Check sheet for the modelled part. Datum: model origin and axes. Units: mm. Face numbers are marked on the shaded views. A direction names the side the tool comes from. Round coordinates to 2 decimals unless told otherwise and drop trailing zeros.
Item 1: Material ranges on line 1 along Y through (x, z) = (0, 5.3); line 2 along Y through (x, z) = (-4, 1.1); line 3 along Y through (x, z) = (3.5, 0.4), recorded low to high.
Item 2: Release check for a two-part mould opening along Y. For the marked faces 1, 2, 3 and 4 record: pulls with the +Y half, pulls with the -Y half, needs draft (parallel to the pull), parting line crosses it, or undercut.
Item 3: Set-up check for the marked faces 5 and 6: record each of +Z, -Z, +X, -X, +Y, -Y from which the full face is reachable in a straight line by a thin tool's end or side.
Item 4: Depth check by flat-ended pin: pin 1 (1.2 mm diameter, centred on x = -3.5, z = 1, fed in from -Y); pin 2 (6 mm diameter, centred on x = -3, y = -5, fed in from -Z); pin 3 (3 mm diameter, centred on y = 5, z = 4, fed in from -X); pin 4 (1.2 mm diameter, centred on y = 4.5, z = 0.5, fed in from -X). Enter the tip coordinate at first touch or a pass-through.
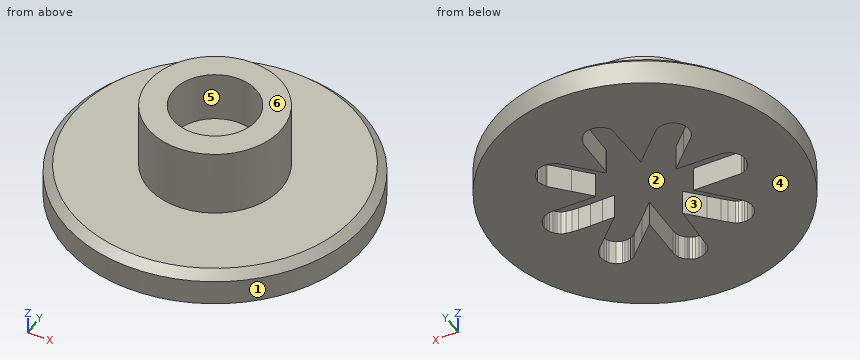
from build123d import *

# Parameters (mm, degrees)
F0_R     = 9
F1_DEPTH = 2
F2_R     = 4
F3_DEPTH = 4
F4_R     = 2.5
F5_DEPTH = 3
F6_SIZE  = 0.5
F8_DEPTH = 1.5


with BuildPart() as f1:
    # F0 (on Top) → F1 (new body)
    with BuildSketch(Plane.XY):
        Circle(F0_R)
    extrude(amount=F1_DEPTH)

    # F2 (on face) → F3 (join)
    with BuildSketch(Plane.XY.offset(2)):
        Circle(F2_R)
    extrude(amount=F3_DEPTH)

    # F4 (on face) → F5 (cut)
    with BuildSketch(Plane.XY.offset(6)):
        Circle(F4_R)
    extrude(amount=-F5_DEPTH, mode=Mode.SUBTRACT)

    # F6
    f6_edges = [f1.edges().sort_by_distance(p)[0] for p in [
        (-9, 0, 2),
    ]]
    chamfer(f6_edges, length=F6_SIZE)

    # F7 (on face) → F8 (cut)
    with BuildSketch(Plane(origin=(0, 0, 0), x_dir=(1, 0, 0), z_dir=(0, 0, -1))):
        Polygon((-0.031379, 5.948377), (-0.235333, 5.919157), (-0.372759, 5.868757), (-0.500818, 5.801363), (-0.64831, 5.683569), (-0.711513, 5.643549), (-0.766303, 5.595223), (-0.884297, 5.389084), (-0.972792, 2.355883), (-1.91674, 3.298237), (-2.464657, 3.842872), (-2.74588, 4.106761), (-3.037677, 4.358384), (-3.197437, 4.424921), (-3.362159, 4.476179), (-3.5244, 4.487041), (-3.686641, 4.476179), (-4.011123, 4.358384), (-4.276609, 4.122796), (-4.349034, 4.030994), (-4.401972, 3.928468), (-4.483097, 3.710516), (-4.483097, 3.357134), (-4.394602, 3.092097), (-4.24711, 2.885957), (-3.303163, 1.914155), (-2.359215, 0.971802), (-5.220556, 0.942353), (-5.397547, 0.883456), (-5.427045, 0.854008), (-5.556038, 0.793243), (-5.614945, 0.756011), (-5.663032, 0.706765), (-5.840022, 0.471176), (-5.958016, 0.117794), (-5.958016, -0.058897), (-5.940408, -0.209293), (-5.899019, -0.353383), (-5.843566, -0.461413), (-5.781025, -0.559523), (-5.655249, -0.699811), (-5.51554, -0.82456), (-5.220556, -0.942354), (-5.075648, -0.968558), (-4.928112, -0.97628), (-4.630589, -0.971802), (-4.188114, -0.971802), (-2.359215, -0.971802), (-2.368134, -1.005446), (-2.388713, -1.030699), (-3.332661, -1.973053), (-4.276609, -2.915406), (-4.34313, -2.999393), (-4.394602, -3.092097), (-4.419005, -3.155066), (-4.453599, -3.209892), (-4.476923, -3.415726), (-4.483097, -3.622171), (-4.464349, -3.757662), (-4.424101, -3.887208), (-4.374765, -3.997645), (-4.306107, -4.093348), (-4.188114, -4.240591), (-4.103985, -4.307), (-4.011123, -4.358385), (-3.71614, -4.476179), (-3.391658, -4.476179), (-3.067176, -4.387833), (-2.890186, -4.240591), (-1.946238, -3.298237), (-1.00229, -2.355884), (-0.884297, -5.418533), (-0.8253, -5.506878), (-0.699524, -5.647167), (-0.559815, -5.771915), (-0.503448, -5.807594), (-0.441821, -5.830812), (-0.341941, -5.885287), (-0.235333, -5.919158), (0.089149, -5.948606), (0.384133, -5.889709), (0.708615, -5.654121), (0.754319, -5.61094), (0.790702, -5.558969), (0.856107, -5.447981), (0.9741, -5.094599), (0.9741, -4.417282), (0.9741, -2.591472), (0.971489, -2.477691), (0.979459, -2.426523), (1.003599, -2.385332), (1.947546, -3.327686), (2.891494, -4.270039), (3.122896, -4.385014), (3.363468, -4.476179), (3.68795, -4.476179), (3.805943, -4.446731), (3.94337, -4.39633), (4.071429, -4.328936), (4.218921, -4.211142), (4.425409, -3.916657), (4.513904, -3.474929), (4.444862, -3.229831), (4.398065, -3.113042), (4.336914, -3.003752), (4.300041, -2.947904), (4.277917, -2.885958), (3.33397, -1.943604), (2.390022, -1.001251), (2.41952, -0.971802), (2.861996, -0.971802), (4.690894, -0.971802), (4.972609, -0.968567), (5.251363, -0.942354), (5.280862, -0.912905), (5.546347, -0.82456), (5.723337, -0.61842), (5.839817, -0.478169), (5.883167, -0.404005), (5.900327, -0.323934), (5.934856, -0.237188), (5.954737, -0.147151), (5.958016, 0.039233), (5.925076, 0.228087), (5.870829, 0.412279), (5.7562, 0.594983), (5.685681, 0.672036), (5.605344, 0.736213), (5.428354, 0.883456), (5.192367, 0.942353), (4.838344, 0.987761), (4.482387, 1.011028), (3.766457, 1.011578), (3.048146, 0.984877), (2.331025, 0.971802), (3.274973, 1.914155), (4.218921, 2.856509), (4.337268, 2.979647), (4.379451, 3.047229), (4.395911, 3.121546), (4.454907, 3.209891), (4.513904, 3.504377), (4.444233, 3.827854), (4.386266, 3.98061), (4.307416, 4.122796), (4.04193, 4.358384), (3.717448, 4.476179), (3.555567, 4.481563), (3.392966, 4.476179), (3.215976, 4.44673), (3.186478, 4.417282), (3.038986, 4.358384), (2.944209, 4.294123), (2.861996, 4.211142), (1.918048, 3.268788), (0.9741, 2.326435), (0.9741, 3.092097), (0.9741, 4.947355), (0.94889, 5.186814), (0.885605, 5.418532), (0.649618, 5.713018), (0.576669, 5.769819), (0.540299, 5.792295), (0.502126, 5.801363), (0.468426, 5.810267), (0.44313, 5.830812), (0.313926, 5.898818), (0.177644, 5.948606), align=None)
    extrude(amount=-F8_DEPTH, mode=Mode.SUBTRACT)


solid = f1.part
Values found:
1. line 1: y = -4 to -2.5, 2.5 to 4
1. line 2: y = -8.06 to -4.36, -2.63 to -0.95, 0.97 to 2.64, 4.36 to 8.06
1. line 3: y = -8.29 to -4.48, -2.14 to -1, 0.97 to 2.11, 4.48 to 8.29
2. face 1: parting line crosses it
2. face 2: undercut
2. face 3: undercut
2. face 4: needs draft
3. face 5: +Z
3. face 6: +Z, +X, -X, +Y, -Y
4. pin 1: stops at y = -8.52
4. pin 2: stops at z = 0
4. pin 3: stops at x = -1.94
4. pin 4: stops at x = -8.11
